For this review, take the finished solid that the model builds, in its own axes (mm). A direction names the side the tool comes from. Give positions to 0.01 mm unless a question says otherwise; leave off trailing zeros. Write each loop counter-clockwise with the first axis right and the second up, starting at its lowest first coordinate (ties: lowest second). Pieces come first, ordered by that corner, then holes.
Q1. We need section A-A (x = 21.5). Write out the cut boundary in (y, z).
Q2. Insertion check: P1, Ø11, axis at x = 28.5, y = -6, coming from the +Z side; P2, Ø11, axis at x = 29.5, y = -6.5, coming from the -Z side. Each pin has a flat end and moves straight along its axis. Give the tip position at first contact, or say it passes through.
Q3. We need section C-C (z = 2.5). Write out the cut boundary in (x, y).
Q4. For line 1 (Y direction, x = 10, z = 1.8); line 2 (X direction, y = 192, z = 3.05); line 3 (Y direction, x = 24.5, z = 2.7), list the stretches that pass through material, from the lowest coordinate up.
Q5. Mouldability with a two-part tool opening along Y and no side actions: class faces 5 (the flat face through (8, 207, 2)), 6 (the flat face through (25, 0, 1)), 7 (the flat face through (0, 129, 2)), 8 (the flat face through (25, 190, 2)) as released by +Y, released by -Y, zero draft, split by the parting line, or undercut.
Q6. We need section B-B (y = 203). Write out the cut boundary in (x, z), then the cut area to 3 significant figures.
Q7. Machinability: for faces 1 (the flat face through (42, 207, 2)), 2 (the flat face through (25, 260, 1.5)), 3 (the flat face through (25, -5, 1.5)), 4 (the flat face through (25, 260, 3.5)), which of the approach directions +Z, -Z, +X, -X, +Y, -Y give a long, thin tool a straight path to every point of the face, cutting with its end or side? Answer none if there is none.
Autodesk Inventor part; units mm, degrees
ref_plane "YZ Plane" through (0, 0, 0) normal (1, 0, 0) x (0, 1, 0)
ref_plane "XZ Plane" through (0, 0, 0) normal (0, 1, 0) x (-1, 0, 0)
ref_plane "XY Plane" through (0, 0, 0) normal (0, 0, 1) x (1, 0, 0)
sketch "Sketch1" plane through (0, 0, 0) normal (0, 0, 1) x (1, 0, 0)
  line L0 (0, 0) -> (50, 0)
  line L1 (50, 0) -> (50, 255.203)
  line L2 (50, 255.203) -> (0, 255.203)
  line L3 (0, 255.203) -> (0, 0)
  line L4 (8, 224) -> (42, 224)
  line L5 (42, 224) -> (42, 190)
  line L6 (42, 190) -> (8, 190)
  line L7 (8, 190) -> (8, 224)
  point P0 (25, 255.203)
  dimension "d0" = 50
  dimension "d1" = 255.203
  dimension "d8" = 34
  dimension "d9" = 34
  dimension "d10" = 8
  dimension "d12" = 190
extrude "Extrusion1" add sketch "Sketch1" along normal blind 5
sketch "Sketch2" plane through (0, 0, 0) normal (0, -1, 0) x (1, 0, 0)
  line L0 (13.5, 2.5) -> (36.5, 2.5) construction
  line L1 (13.5, 1.5) -> (36.5, 1.5)
  line L2 (36.5, 3.5) -> (13.5, 3.5)
  arc A0 (13.5, 3.5) -> (13.5, 1.5) centre (13.5, 2.5) ccw
  arc A1 (36.5, 1.5) -> (36.5, 3.5) centre (36.5, 2.5) ccw
  line L3 (0, 5) -> (50, 5)
  point P0 (0, 0)
  point P1 (25, 2.5)
  point P2 (37.5, 2.5)
  point P3 (12.5, 2.5)
  dimension "d13" = 2
  dimension "d21" = 25
  dimension "d22" = 25
  dimension "d23" = 2.5
extrude "Extrusion2" add sketch "Sketch2" along normal blind 10
sketch "Sketch4" plane through (0, 255.203, 0) normal (0, 1, 0) x (1, 0, 0)
  line L0 (36.5, -2.5) -> (13.5, -2.5) construction
  line L1 (36.5, -1.5) -> (13.5, -1.5)
  line L2 (13.5, -3.5) -> (36.5, -3.5)
  arc A0 (36.5, -3.5) -> (36.5, -1.5) centre (36.5, -2.5) ccw
  arc A1 (13.5, -1.5) -> (13.5, -3.5) centre (13.5, -2.5) ccw
  point P0 (0, 0)
  point P1 (25, -2.5)
  point P2 (12.5, -2.5)
  point P3 (37.5, -2.5)
  dimension "d24" = 2
  dimension "d26" = 25
  dimension "d28" = 2.5
  dimension "d29" = 25
extrude "Extrusion3" add sketch "Sketch4" along normal blind 10
properties part number "partttt"
Computed:
1. outline: (-10, 1.5) - (0, 1.5) - (0, 0) - (190, 0) - (190, 5) - (0, 5) - (0, 3.5) - (-10, 3.5) - close; (224, 0) - (255.2, 0) - (255.2, 1.5) - (265.2, 1.5) - (265.2, 3.5) - (255.2, 3.5) - (255.2, 5) - (224, 5) - close
2. P1: stops at z = 3.5
2. P2: stops at z = 1.5
3. outline: (0, 0) - (12.5, 0) - (12.5, -10) - (37.5, -10) - (37.5, 0) - (50, 0) - (50, 255.2) - (37.5, 255.2) - (37.5, 265.2) - (12.5, 265.2) - (12.5, 255.2) - (0, 255.2) - close; hole (8, 190) - (42, 190) - (42, 224) - (8, 224) - close
4. line 1: y = 0 to 190, 224 to 255.2
4. line 2: x = 0 to 8, 42 to 50
4. line 3: y = -10 to 190, 224 to 265.2
5. face 5: undercut
5. face 6: released by -Y
5. face 7: zero draft
5. face 8: undercut
6. outline: (0, 0) - (8, 0) - (8, 5) - (0, 5) - close; (42, 0) - (50, 0) - (50, 5) - (42, 5) - close
6. area: 80.0 mm2
7. face 1: +Z, -Z
7. face 2: -Z, +X, -X, +Y
7. face 3: -Z, +X, -X, -Y
7. face 4: +Z, +X, -X, +Y
